Here's how the part is built. I have some questions about the finished solid (model axes, mm). Coordinates: 2 decimals unless noted, no trailing zeros. Write each loop counter-clockwise with the first axis right and the second up, starting at its lowest first coordinate (ties: lowest second). Pieces come first, ordered by that corner, then holes. Notation, with made-up numbers: M 88,88 L 145,88 A32 cw 145,117 Z; hole C 44.5,46 d2. An arc over 180 degrees is marked long. Use a Markdown table: item, result.
```python
from build123d import *

# Parameters (mm, degrees)
SKETCH1_R           = 1.4732
SKETCH1_R_2         = 4.7625
BOSS_EXTRUDE1_DEPTH = 6.35


with BuildPart() as part:
    # Sketch1 → Boss-Extrude1 (new body)
    with BuildSketch(Plane.XY):
        with BuildLine():
            Line((0, 0), (0, 101.854))
            ThreePointArc((0, 101.854), (1.859871939, 106.344128061), (6.35, 108.204))
            Line((6.35, 108.204), (158.75, 108.204))
            ThreePointArc((158.75, 108.204), (163.240128061, 106.344128061), (165.1, 101.854))
            Line((165.1, 101.854), (165.1, 0))
            Line((165.1, 0), (0, 0))
        make_face()
        with Locations((6.35, 6.35)):
            Circle(SKETCH1_R, mode=Mode.SUBTRACT)
        with Locations((158.75, 6.35)):
            Circle(SKETCH1_R, mode=Mode.SUBTRACT)
        with Locations((158.75, 101.854)):
            Circle(SKETCH1_R, mode=Mode.SUBTRACT)
        with Locations((6.35, 101.854)):
            Circle(SKETCH1_R, mode=Mode.SUBTRACT)
        with Locations((82.55, 82.804)):
            Circle(SKETCH1_R_2, mode=Mode.SUBTRACT)
    extrude(amount=BOSS_EXTRUDE1_DEPTH)


solid = part.part
```
1. Will this pin go through, and if not, where does the flat tip stop? pin 1 Ø2.5 at (x, y) = (6.35, 101.854) entering from -Z (3 decimals).
Answers follow:
| item | result |
|---|---|
| pin 1 | passes through |
2. We'd pull the mould along X, two halves only. Please class faces 1 (the face through (163.19, 106.393, 3.131)), 2 (the face through (77.79, 83.01, 3.13)), 3 (the face through (1.811, 106.294, 3.131)), 4 (the face through (84, 0, 3)): +X half, -X half, draft (parallel to the pull), parting line (faces both ways), or undercut.
Answers follow:
| item | result |
|---|---|
| face 1 | +X half |
| face 2 | undercut |
| face 3 | -X half |
| face 4 | draft |
3. I need wall thicknesses on probe 1 along Y at (x, z) = (158.75, 1.75); probe 2 along Y at (x, z) = (82, 4.75); probe 3 along Y at (x, z) = (82.55, 3). Which ranges of each line are inside material? Lowest first, please.
Answers follow:
| item | result |
|---|---|
| probe 1 | y = 0 to 4.88, 7.82 to 100.38, 103.33 to 108.2 |
| probe 2 | y = 0 to 78.07, 87.53 to 108.2 |
| probe 3 | y = 0 to 78.04, 87.57 to 108.2 |
4. Suppose I cut it at A-A on x = 82.55. Write out the boundary of the cut face in (y, z).
Answers follow:
| item | result |
|---|---|
| outline | M 0,0 L 78.04,0 L 78.04,6.35 L 0,6.35 Z; M 87.57,0 L 108.2,0 L 108.2,6.35 L 87.57,6.35 Z |
